Drawing for the job (mm, zero at the part's lowest x, y, z). Give positions to 0.01 mm unless a question says otherwise; leave off trailing zeros. Order: outer loops, then holes, each group sorted by start corner. A loop starts at its lowest first (then second) coordinate and runs counter-clockwise, first axis right, second up. Notation, with made-up numbers: (0.25, 40.5) - (49.25, 40.5) arc R19 cw to (49.25, 55.5) - close; hole circle Ø8 at (72.5, 65). An arc over 180 degrees is marked (long way). One line per item, written item: value.
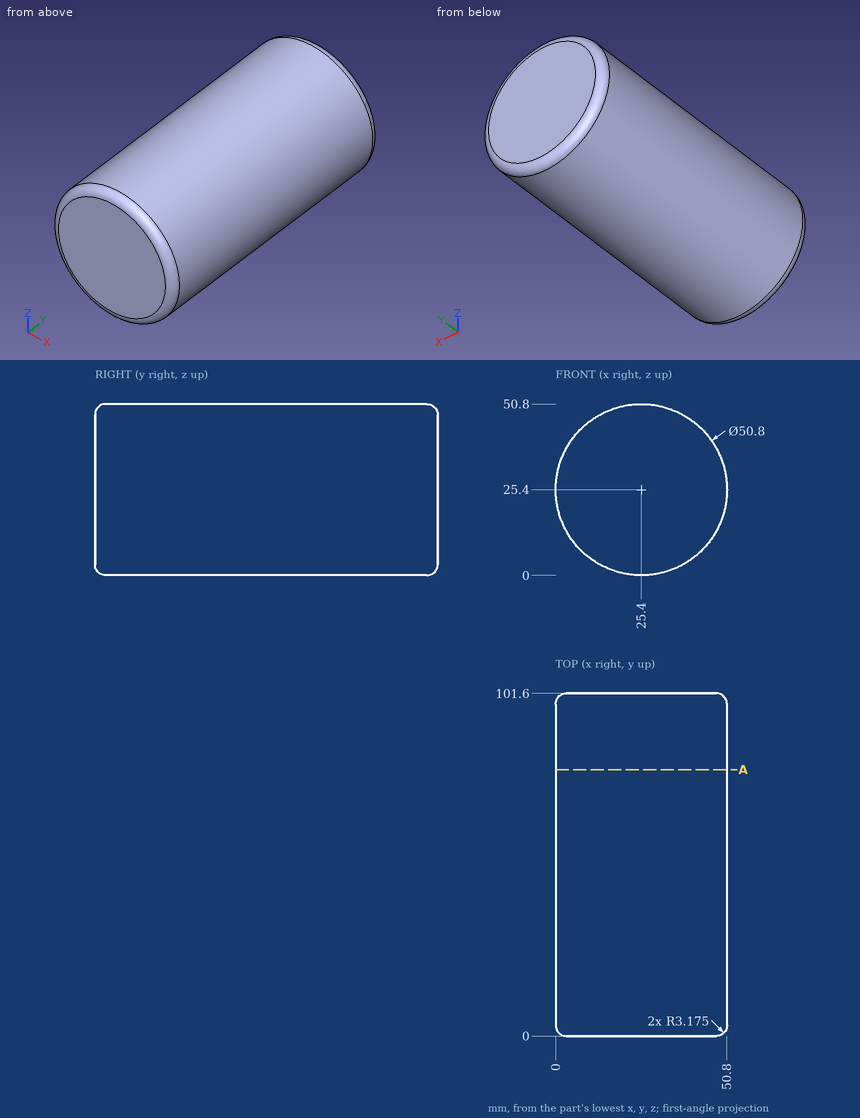
1) Drill centre lines: line 1 along X through (y, z) = (95, 26); line 2 along X through (y, z) = (5.5, 16); line 3 along Z through (x, y) = (7.5, 97). Where is each one in solid material? Low to high. Write a range as from..to.
Outcome:
line 1: x = 0.01..50.79
line 2: x = 1.8..49
line 3: z = 7.38..43.42
2) Cut at A-A, the plane y = 79. Give the cut face in (x, z).
Outcome:
outline: circle Ø50.8 at (25.4, 25.4)
3) Pin check, flat tips, straight feed: pin 1 (8 mm diameter, centred on y = 25, z = 43.5, fed in from -X); pin 2 (10 mm diameter, centred on y = 46, z = 45.5, fed in from +X); pin 3 (8 mm diameter, centred on x = 39, y = 74.5, fed in from -Z). Stop position of each tip, or through.
Outcome:
pin 1: stops at x = 4.27
pin 2: stops at x = 45.82
pin 3: stops at z = 1.88
